```python
from build123d import *

# Parameters (mm, degrees)
BOSS_EXTRUDE1_DEPTH = 10
CHAMFER1_SIZE       = 2
CUT_EXTRUDE1_DEPTH  = 5
SKETCH5_R           = 34.202431596
SKETCH5_R_2         = 6
CUT_EXTRUDE2_DEPTH  = 2
CUT_EXTRUDE3_DEPTH  = 4
CHAMFER2_SIZE       = 0.5
SKETCH7_W           = 40.92273168
SKETCH7_H           = 22.154300558
SKETCH7_R           = 4
CUT_EXTRUDE4_DEPTH  = 0.5
CHAMFER3_SIZE       = 0.5


# Some blends are built 0.0001 mm under size
with BuildPart() as part:
    # Sketch1 → Boss-Extrude1 (new body)
    with BuildSketch(Plane(origin=(0, 0, 0), x_dir=(1, 0, 0), z_dir=(0, 1, 0))):
        with BuildLine():
            Line((0, 6), (19, 6))
            ThreePointArc((19, 6), (25, 0), (19, -6))
            Line((19, -6), (0, -6))
            ThreePointArc((0, -6), (-6, 0), (0, 6))
        make_face()
    extrude(amount=BOSS_EXTRUDE1_DEPTH)

    # Sketch2 → Cut-Revolve1 (revolve, cut)
    with BuildSketch(Plane.XY, mode=Mode.PRIVATE) as cut_revolve1_sk:
        Polygon((0, 10), (-2.55, 10), (-2.55, 5), (-2.1, 5), (-2.1, 2), (-2.55, 2), (-2.55, 0), (0, 0), align=None)
    revolve(cut_revolve1_sk.sketch.rotate(Axis((0, 0, 0), (0, 1, 0)), 270), axis=Axis((0, 0, 0), (0, 1, 0)), mode=Mode.SUBTRACT)

    # Sketch3 → Cut-Revolve2 (revolve, cut)
    with BuildSketch(Plane.XY, mode=Mode.PRIVATE) as cut_revolve2_sk:
        Polygon((19, 10), (16.5, 10), (16.5, 6), (16.925, 6), (16.925, 0), (19, 0), align=None)
    revolve(cut_revolve2_sk.sketch.rotate(Axis((19, 0, 0), (0, 1, 0)), 270), axis=Axis((19, 0, 0), (0, 1, 0)), mode=Mode.SUBTRACT)

    # Chamfer1
    chamfer1_edges = [part.edges().sort_by_distance(p)[0] for p in [
        (25, 10, 0),
        (9.5, 10, -6),
        (-6, 10, 0),
        (9.5, 10, 6),
    ]]
    chamfer(chamfer1_edges, length=CHAMFER1_SIZE)

    # Sketch4 → Cut-Extrude1 (cut)
    with BuildSketch(Plane.XZ):
        Polygon((2.107328483, 3.65), (-2.107328483, 3.65), (-4.214656965, 0), (-2.107328483, -3.65), (2.107328483, -3.65), (4.214656965, 0), align=None)
    extrude(amount=-CUT_EXTRUDE1_DEPTH, mode=Mode.SUBTRACT)

    # Sketch5 → Cut-Extrude2 (cut)
    with BuildSketch(Plane.XZ):
        Circle(SKETCH5_R)
        with Locations(Location((0, 0, 0), (0, 0, 90))):
            Circle(SKETCH5_R_2, mode=Mode.SUBTRACT)
    extrude(amount=-CUT_EXTRUDE2_DEPTH, mode=Mode.SUBTRACT)

    # Sketch6 → Cut-Extrude3 (cut)
    with BuildSketch(Plane(origin=(0, 10, 0), x_dir=(1, 0, 0), z_dir=(0, 1, 0))):
        Polygon((20.674315781, -2.9), (22.348631561, 0), (20.674315781, 2.9), (17.325684219, 2.9), (15.651368439, 0), (17.325684219, -2.9), align=None)
    extrude(amount=-CUT_EXTRUDE3_DEPTH, mode=Mode.SUBTRACT)

    # Chamfer2
    # the kernel refuses this chamfer: 0.5 mm, written as the material it takes off along each edge
    with BuildSketch(Plane(origin=(19, 2, 0), x_dir=(0, 0, -1), z_dir=(-1, 0, 0))) as chamfer2_piece_1:
        Polygon((6 - CHAMFER2_SIZE, 0), (6, -CHAMFER2_SIZE), (6, 0), align=None)
    revolve(axis=Axis((19, 2, 0), (0, -1, 0)), revolution_arc=180, mode=Mode.SUBTRACT)
    with BuildSketch(Plane(origin=(-1.285841494, 2, 6), x_dir=(0, -0.02749587661058651, -0.9996219169112968), z_dir=(1, 0, 0))) as chamfer2_piece_2_section:
        Polygon((CHAMFER2_SIZE * 0.999621916911, CHAMFER2_SIZE * 0.0274958766106), (-CHAMFER2_SIZE * 0.0274958766106, CHAMFER2_SIZE * 0.999621916911), (0, 0), align=None)
    chamfer2_piece_2 = extrude(amount=20.285841494, mode=Mode.PRIVATE)
    chamfer2_piece_2 = chamfer2_piece_2 - Plane(origin=(0, 2.170377839, 0), x_dir=(0, 0, 1), z_dir=(0, -1, 0)) * Cylinder(6, 43, mode=Mode.PRIVATE)
    add(chamfer2_piece_2, mode=Mode.SUBTRACT)
    with BuildSketch(Plane(origin=(19, 2, -6), x_dir=(0, 0.9996219169112968, -0.027495876610585623), z_dir=(-1, 0, 0))) as chamfer2_piece_3_section:
        Polygon((CHAMFER2_SIZE * 0.999621916911, -CHAMFER2_SIZE * 0.0274958766106), (-CHAMFER2_SIZE * 0.0274958766106, -CHAMFER2_SIZE * 0.999621916911), (0, 0), align=None)
    chamfer2_piece_3 = extrude(amount=20.285841494, mode=Mode.PRIVATE)
    chamfer2_piece_3 = chamfer2_piece_3 - Plane(origin=(0, 2.17037784, 0), x_dir=(0, 0, 1), z_dir=(0, -1, 0)) * Cylinder(6, 43, mode=Mode.PRIVATE)
    add(chamfer2_piece_3, mode=Mode.SUBTRACT)

    # Sketch7 → Cut-Extrude4 (cut)
    with BuildSketch(Plane(origin=(0, 10, 0), x_dir=(1, 0, 0), z_dir=(0, 1, 0))):
        with Locations((9.45107525, -1.501135351)):
            Rectangle(SKETCH7_W, SKETCH7_H)
        with Locations(Location((19, 0, 0), (0, 0, 270))):
            Circle(SKETCH7_R, mode=Mode.SUBTRACT)
        with Locations(Location((0, 0, 0), (0, 0, 270))):
            Circle(SKETCH7_R, mode=Mode.SUBTRACT)
    extrude(amount=-CUT_EXTRUDE4_DEPTH, mode=Mode.SUBTRACT)

    # Chamfer3
    chamfer3_edges = [part.edges().sort_by_distance(p)[0] for p in [
        (0, 9.5, -4),
        (19, 9.5, -4),
    ]]
    chamfer(chamfer3_edges, length=CHAMFER3_SIZE - 0.0001)  # a hair under: the kernel refuses the full size


solid = part.part
```
Could you check a few things on this model? Use its own coordinates, in mm. A direction names the side the tool comes from. Give positions to 0.01 mm unless a question says otherwise; leave off trailing zeros. Answer in a Markdown table with one row per item. Add a question column.
Q1. We'd pull the mould along Z, two halves only. Please class faces 1 (the face through (0, 10, 3)), 2 (the face through (24, 9, 0)), 3 (the face through (19, 8, 2.9)): +Z half, -Z half, draft (parallel to the pull), parting line (faces both ways), or undercut.
Q2. Please list where these lines run through material, in increasing order: L1, parallel to X at y = 5.15, z = 0 (3 decimals); L2, parallel to Z at x = 19, y = 7.75; L3, parallel to Y at x = 13.5, z = 3.5. Write a range as from..to.
Q3. For pin 1 (2.5 mm diameter, centred on x = 19, z = 0, fed in from +Y); pin 2 (6.5 mm diameter, centred on x = 0, z = 0, fed in from -Y); pin 3 (3 mm diameter, centred on x = 6.5, z = -2.5, fed in from +Y); pin 4 (1 mm diameter, centred on y = 2.5, z = -3, fed in from +X), each with a flat end and sliding along its axis, tell me the tip position at first contact or that it passes through.
Q4. If we section it at A-A (z = -1): State how many separate pieces and enclosed holes the cut face has, plus the area to 3 significant figures.
Q5. Which directions (+Z, -Z, +X, -X, +Y, -Y) give clear straight access to the entire face, cutting with the end or side of a thin tool? Please do faces 4 (the face through (-0.77, 7.46, -2.43)), 5 (the face through (21.523, 8.028, -1.43)), 6 (the face through (0, 2, 3.65)).
The answers:
| question | item | result |
|---|---|---|
| 1 | face 1 | draft |
| 1 | face 2 | parting line |
| 1 | face 3 | undercut |
| 2 | L1 | x = -6..-2.55, 2.55..16.925, 21.075..25 |
| 2 | L2 | z = -6..-2.9, 2.9..6 |
| 2 | L3 | y = 2..9.5 |
| 3 | pin 1 | passes through |
| 3 | pin 2 | stops at y = 5 |
| 3 | pin 3 | stops at y = 9.5 |
| 3 | pin 4 | stops at x = 24.45 |
| 4 | separate pieces | 3 |
| 4 | enclosed holes | 0 |
| 4 | area | 164 mm^2 |
| 5 | face 4 | +Y, -Y |
| 5 | face 5 | +Y |
| 5 | face 6 | -Y |
